```python
from build123d import *

# Parameters (mm, degrees)
F0_R     = 17.5
F1_DEPTH = 33
F2_R     = 22.5
F3_DEPTH = 4
F4_R     = 7.5
F4_R_2   = 4.075
F5_DEPTH = 7.7
F6_DEPTH = 37.001
F7_SIZE  = 2
F8_SIZE  = 0.5


with BuildPart() as f1:
    # F0 (on Top) → F1 (new body)
    with BuildSketch(Plane.XY):
        Circle(F0_R)
    extrude(amount=F1_DEPTH)

    # F2 (on face) → F3 (join)
    with BuildSketch(Plane.XY.offset(33)):
        Circle(F2_R)
    extrude(amount=F3_DEPTH)

    # F4 (on face) → F5 (cut)
    with BuildSketch(Plane.XY.offset(37)):
        with Locations((-8.8, 0)):
            Circle(F4_R)
        with Locations((-8.8, 0)):
            Circle(F4_R_2, mode=Mode.SUBTRACT)
        with Locations((8.8, 0)):
            Circle(F4_R)
        with Locations((8.8, 0)):
            Circle(F4_R_2, mode=Mode.SUBTRACT)
    extrude(amount=-F5_DEPTH, mode=Mode.SUBTRACT)

    # F6 (cut, through all): faces of the model
    f6_faces = [f1.faces().sort_by_distance(p)[0] for p in [
        (-8.8, 0, 37),
        (8.8, 0, 37),
    ]]
    extrude(f6_faces, amount=-F6_DEPTH, mode=Mode.SUBTRACT)

    # F7
    f7_edges = [f1.edges().sort_by_distance(p)[0] for p in [
        (-22.5, 0, 37),
    ]]
    chamfer(f7_edges, length=F7_SIZE)

    # F8
    f8_edges = [f1.edges().sort_by_distance(p)[0] for p in [
        (-16.3, 0, 37),
        (1.3, 0, 37),
        (-12.875, 0, 0),
        (4.725, 0, 0),
    ]]
    chamfer(f8_edges, length=F8_SIZE)


solid = f1.part
```
Read the model definition and answer for the solid it produces. Units are mm, in the model's axes. A direction names the side the tool comes from. Round coordinates to 2 decimals unless told otherwise and drop trailing zeros. Write each loop counter-clockwise with the first axis right and the second up, starting at its lowest first coordinate (ties: lowest second). Pieces come first, ordered by that corner, then holes. Notation, with made-up numbers: (37.25, 80.25) -> (61.25, 80.25) arc R29 cw to (61.25, 108.25) -> close; hole circle Ø9 at (-27.5, 65.25). An arc over 180 degrees is marked (long way). Answer in a Markdown table with one row per item. Add a question column.
1) Which of the six approach directions +Z, -Z, +X, -X, +Y, -Y give full straight-line access (tool end or side, diameter ignored) to faces 4 (the face through (12, -13, 33)), 5 (the face through (-5.6, -3.2, 29.3)), 6 (the face through (0, 0, 0))?
2) Find section A-A, the plane y = 0. State how many separate pieces and enclosed holes the cut face has, and give its area (3 significant figures).
3) Consider line 1 (Z direction, x = -19.5, y = -6); line 2 (Z direction, x = -4, y = -2.5); line 3 (X direction, y = -3, z = 13). Determine where each line is inside the solid, lowest interval first.
4) Determine the mould class of faces 1 (the face through (-12.034, -2.48, 15.102)), 2 (the face through (0, 0, 37)), 3 (the face through (10.382, -19.961, 33.986)) for opening direction X: pulls with the +X half, pulls with the -X half, needs draft (parallel to the pull), parting line crosses it, or undercut.
5) Given P1, Ø5, axis at y = -16, z = 16, coming from the +X side; P2, Ø7.5, axis at x = 8.8, y = 0, coming from the +Z side; P3, Ø4, axis at y = 11.5, z = 24, coming from the +X side; P4, Ø3, axis at x = -2.5, z = 14.5, coming from the +Y side, each flat-ended and moving along its own axis, determine where each tip first touches the part or whether it passes through.
6) Find section C-C, the plane z = 8. Determine the outline of the cut face in (x, y) (3 decimals), and give its area (3 significant figures).
7) Find section B-B, the plane x = 0. Determine the outline of the cut face in (y, z), and give its area (3 significant figures).
Findings below:
| question | item | result |
|---|---|---|
| 1 | face 4 | -Z |
| 1 | face 5 | +Z |
| 1 | face 6 | -Z, +X, -X, +Y, -Y |
| 2 | separate pieces | 3 |
| 2 | enclosed holes | 0 |
| 2 | area | 621 mm² |
| 3 | line 1 | 33 to 37 |
| 3 | line 2 | 0 to 29.3 |
| 3 | line 3 | -17.24 to -11.56, -6.04 to 6.04, 11.56 to 17.24 |
| 4 | face 1 | undercut |
| 4 | face 2 | needs draft |
| 4 | face 3 | parting line crosses it |
| 5 | P1 | x = 11.14 |
| 5 | P2 | through |
| 5 | P3 | x = 14.7 |
| 5 | P4 | y = 17.47 |
| 6 | outline | circle Ø35 at (0, 0); hole circle Ø8.15 at (-8.8, 0); hole circle Ø8.15 at (8.8, 0) |
| 6 | area | 858 mm² |
| 7 | outline | (-22.5, 33) -> (-17.5, 33) -> (-17.5, 0) -> (17.5, 0) -> (17.5, 33) -> (22.5, 33) -> (22.5, 35) -> (20.5, 37) -> (-20.5, 37) -> (-22.5, 35) -> close |
| 7 | area | 1,330 mm² |
